```python
from build123d import *

# Parameters (mm, degrees)
SKETCH_2_W      = 79.3
SKETCH_2_H      = 5.45
SKETCH_2_W_2    = 5.45
SKETCH_2_H_2    = 29.65
EXTRUDE_1_DEPTH = 6


with BuildPart() as part:
    # Эскиз2 → Бобышка-Вытянуть1 (new body)
    with BuildSketch(Plane.XY):
        Polygon((0, 0), (-29.3, 0), (-29.3, 5.45), (0, 5.45), (0, 15.8), (-5.45, 15.8), (-5.45, 45.1), (0, 45.1), (0, 55.45), (-29.3, 55.45), (-29.3, 60.9), (-59.3, 60.9), (-59.3, 55.45), (-140, 55.45), (-140, 60.9), (-170, 60.9), (-170, 55.45), (-200, 55.45), (-200, 5.45), (-170, 5.45), (-170, 0), (-200, 0), (-200, -250), (-170, -250), (-170, -255.45), (-140, -255.45), (-140, -250), (-59.3, -250), (-59.3, -255.45), (-29.3, -255.45), (-29.3, -250), (0, -250), (0, -235), (-5.45, -235), (-5.45, -205.35), (0, -205.35), (0, -175), (-5.45, -175), (-5.45, -145.35), (0, -145.35), (0, -115), (-5.45, -115), (-5.45, -85.35), (0, -85.35), align=None)
        with Locations((-99.65, 2.725)):
            Rectangle(SKETCH_2_W, SKETCH_2_H, mode=Mode.SUBTRACT)
        with Locations((-71.175, -220.175)):
            Rectangle(SKETCH_2_W_2, SKETCH_2_H_2, mode=Mode.SUBTRACT)
        with Locations((-71.175, -160.175)):
            Rectangle(SKETCH_2_W_2, SKETCH_2_H_2, mode=Mode.SUBTRACT)
    extrude(amount=EXTRUDE_1_DEPTH)


solid = part.part
```
Verification items for the finished model (mm, model axes). A direction names the side the tool comes from. Give positions to 0.01 mm unless a question says otherwise; leave off trailing zeros. Order: outer loops, then holes, each group sorted by start corner. A loop starts at its lowest first (then second) coordinate and runs counter-clockwise, first axis right, second up. Notation, with made-up numbers: (-10.75, 48.25) - (30.25, 48.25) arc R15 cw to (30.25, 71.25) - close; hole circle Ø4 at (56.5, -24). An arc over 180 degrees is marked (long way). Answer as CSV lines item,"result". Start each with the question number.
Item 1: Section check B-B, the plane z = 4.25. State how many separate pieces and enclosed holes the cut face has, plus the area to 3 significant figures.
Item 2: Access from +Z, -Z, +X, -X, +Y, -Y to the whole of each face (thin tool, end or side, straight path). Record for faces 1 (the face through (-5.45, -220, 3)), 2 (the face through (-185, 55.45, 3)), 3 (the face through (-15, -250, 3)).
Item 3: Material ranges on L1, parallel to Y at x = -20, z = 4.9; L2, parallel to X at y = -166.5, z = 5.45; L3, parallel to X at y = 22, z = 5.4, recorded low to high.
Item 4: Gauge pin test, flat ends, axial feed: pin 1 (1.8 mm diameter, centred on x = -18.5, z = 2.5, fed in from -Y); pin 2 (1.5 mm diameter, centred on x = -66.5, y = 18, fed in from -Z); pin 3 (1.6 mm diameter, centred on x = -71, z = 3, fed in from +Y); pin 4 (2.5 mm diameter, centred on y = 57.5, z = 2, fed in from +X). Record the tip position at first contact, or that the pin passes through.
Item 5: Mould release check, pull along X, two halves, no side actions. Record for faces 4 (the face through (-99, 55.45, 3)), 5 (the face through (-155, 60.9, 3)), 6 (the face through (0, 11, 3)): released by +X, released by -X, zero draft, split by the parting line, or undercut.
Item 6: Section check A-A, the plane x = -127. Record the boundary of the cut face in (y, z).
Filled in:
1,separate pieces,"1"
1,enclosed holes,"3"
1,area,"60,000 mm^2"
2,face 1,"+Z, -Z, +X"
2,face 2,"+Z, -Z, -X, +Y"
2,face 3,"+Z, -Z, +X, -Y"
3,L1,"-250 to 0, 5.45 to 55.45"
3,L2,"-200 to -73.9, -68.45 to -5.45"
3,L3,"-200 to -5.45"
4,pin 1,"y = -250"
4,pin 2,"z = 0"
4,pin 3,"y = 55.45"
4,pin 4,"x = -29.3"
5,face 4,"undercut"
5,face 5,"zero draft"
5,face 6,"released by +X"
6,outline,"(-250, 0) - (0, 0) - (0, 6) - (-250, 6) - close; (5.45, 0) - (55.45, 0) - (55.45, 6) - (5.45, 6) - close"
